CAD build for the part. Positions are in the model's coordinates, mm. Round coordinates to 2 decimals unless told otherwise and drop trailing zeros. Order: outer loops, then holes, each group sorted by start corner. A loop starts at its lowest first (then second) coordinate and runs counter-clockwise, first axis right, second up. Notation, with made-up numbers: M 83,25 L 120,25 A31 ccw 120,49 Z; hole C 24.25,82 d8. An arc over 180 degrees is marked long. Put each result on its own line as item: value.
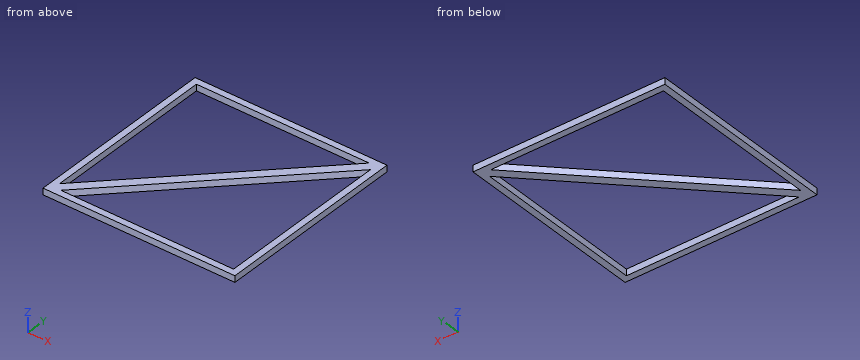
```python
from build123d import *

# Parameters (mm, degrees)
F0_W     = 300
F0_H     = 300
F1_DEPTH = 10


with BuildPart() as f1:
    # F0 (on Top) → F1 (new body)
    with BuildSketch(Plane.XY):
        with Locations((150, 150)):
            Rectangle(F0_W, F0_H)
        Polygon((20, 10), (290, 280), (290, 10), align=None, mode=Mode.SUBTRACT)
        Polygon((10, 290), (280, 290), (10, 20), align=None, mode=Mode.SUBTRACT)
    extrude(amount=F1_DEPTH)


solid = f1.part
```
Item 1: Band-saw the part on B-B on z = 6. Give the cut face in (x, y).
Answers below:
outline: M 0,0 L 300,0 L 300,300 L 0,300 Z; hole M 10,20 L 280,290 L 10,290 Z; hole M 20,10 L 290,10 L 290,280 Z
Item 2: Band-saw the part on A-A on x = 235. Give the cut face in (y, z), and give its area (3 significant figures).
Answers below:
outline: M 0,0 L 10,0 L 10,10 L 0,10 Z; M 225,0 L 245,0 L 245,10 L 225,10 Z; M 290,0 L 300,0 L 300,10 L 290,10 Z
area: 400 mm²
Item 3: Probe line 1 along X through (y, z) = (196.5, 1); line 2 along Y through (x, z) = (191, 3); line 3 along X through (y, z) = (38.5, 5.5). List the from-to ranges inside material, lowest first. Write a range as [from, to].
Answers below:
line 1: [0, 10], [186.5, 206.5], [290, 300]
line 2: [0, 10], [181, 201], [290, 300]
line 3: [0, 10], [28.5, 48.5], [290, 300]
Item 4: Band-saw the part on C-C on y = 171. Give the cut face in (x, z).
Answers below:
outline: M 0,0 L 10,0 L 10,10 L 0,10 Z; M 161,0 L 181,0 L 181,10 L 161,10 Z; M 290,0 L 300,0 L 300,10 L 290,10 Z
